Work out the finished part from the listing and answer in its coordinate system (mm). Round coordinates to 2 decimals unless told otherwise and drop trailing zeros. Loops run counter-clockwise (first coordinate to the right, second up) from the corner with the lowest first, then second, coordinate; pieces in that order, holes last. Notation, with made-up numbers: (-6.5, -1.75) - (14.5, -1.75) arc R30 ccw to (14.5, 26.25) - close; hole circle Ø1 at (61.5, 7.25). An arc over 180 degrees is marked (long way). Answer as CSV lines item,"result". Start each with the question number.
Q1. The mould has two halves that part along X. Classify faces 1 (the face through (7.2, -4.1, 2.3)), 2 (the face through (-2, 6, 2.5)), 3 (the face through (-1.08, -4.88, -0.02)): +X half, -X half, draft (parallel to the pull), parting line (faces both ways), or undercut.
Q2. Each of these flat-tipped pins is pushed along its axis until it touches: pin 1 Ø2 at (x, z) = (-2.5, 1) entering from +Y; pin 2 Ø3 at (x, z) = (-5, -1.5) entering from +Y; pin 3 Ø5 at (x, y) = (-2.5, 2) entering from -Z; pin 4 Ø6 at (x, y) = (0, 0) entering from +Z. Where does it stop, or does it pass through?
Q3. Section A-A on z = 1.1 is taken. Write down the section's boundary in (x, y).
Q4. Straight lines are drawn through the part: L1, parallel to X at y = 4.75, z = 1.85; L2, parallel to X at y = -3.5, z = -1.25; L3, parallel to Y at x = 3.75, z = 1.45. For each, find the intervals that lie inside material, in ascending order. Write a range as [from, to].
```python
from build123d import *

# Parameters (mm, degrees)
SKETCH1_R           = 5
BOSS_EXTRUDE1_DEPTH = 2.5
SKETCH2_OUTSIDE_W   = 40.128
SKETCH2_OUTSIDE_H   = 42.604
SKETCH2_OUTSIDE_R   = 8
CUT_EXTRUDE1_DEPTH  = 6
CUT_EXTRUDE1_TAPER  = 55
CHAMFER1_SIZE       = 1


with BuildPart() as part:
    # Sketch1 → Boss-Extrude1 (new body, symmetric)
    with BuildSketch(Plane.XY):
        Polygon((-8, 4.618802154), (-8, -4.618802154), (0, -9.237604307), (8, -4.618802154), (8, 4.618802154), (0, 9.237604307), align=None)
        Circle(SKETCH1_R, mode=Mode.SUBTRACT)
    extrude(amount=BOSS_EXTRUDE1_DEPTH, both=True)

    # Sketch2 outside → Cut-Extrude1 (cut, through all)
    with BuildSketch(Plane.XY.offset(2.5)):
        Rectangle(SKETCH2_OUTSIDE_W, SKETCH2_OUTSIDE_H)
        Circle(SKETCH2_OUTSIDE_R, mode=Mode.SUBTRACT)
    cut_extrude1 = extrude(amount=-CUT_EXTRUDE1_DEPTH, taper=CUT_EXTRUDE1_TAPER, mode=Mode.SUBTRACT)

    # Mirror1: Cut-Extrude1 across plane
    add(cut_extrude1.mirror(Plane.XY), mode=Mode.SUBTRACT)

    # Chamfer1
    chamfer1_edges = [part.edges().sort_by_distance(p)[0] for p in [
        (-5, 0, -2.5),
        (-5, 0, 2.5),
    ]]
    chamfer(chamfer1_edges, length=CHAMFER1_SIZE)


solid = part.part
```
Findings:
1,face 1,"+X half"
1,face 2,"draft"
1,face 3,"undercut"
2,pin 1,"stops at y = 8.37"
2,pin 2,"stops at y = 7.22"
2,pin 3,"stops at z = -2.2"
2,pin 4,"passes through"
3,outline,"(-8, -4.62) - (0, -9.24) - (8, -4.62) - (8, 4.62) - (0, 9.24) - (-8, 4.62) - close; hole circle Ø10 at (0, 0)"
4,L1,"x = [-7.56, -2.46], [2.46, 7.56]"
4,L2,"x = [-8, -3.57], [3.57, 8]"
4,L3,"y = [-7.07, -3.31], [3.31, 7.07]"
